from build123d import *

# Parameters (mm, degrees)
EXTRUDE_1_DEPTH     = 20
SKETCH_2_R          = 1.5
CUT_EXTRUDE_1_DEPTH = 20


with BuildPart() as part:
    # 草图1 → 凸台-拉伸1 (new body)
    with BuildSketch(Plane.XY):
        with BuildLine():
            Line((-3, 20), (-3, 10.583005244))
            ThreePointArc((-3, 10.583005244), (-11, 0), (-3, -10.583005244))
            Line((-3, -10.583005244), (-3, -45.2))
            Line((-3, -45.2), (0, -45.2))
            Line((0, -45.2), (0, -10))
            ThreePointArc((0, -10), (-10, 0), (0, 10))
            Line((0, 10), (0, 20))
            Line((0, 20), (-3, 20))
        make_face()
    extrude(amount=EXTRUDE_1_DEPTH)

    # 草图2 → 切除-拉伸1 (cut)
    with BuildSketch(Plane.ZY.offset(3)):
        with Locations((5, 15.291502622)):
            Circle(SKETCH_2_R)
        with Locations((15, 15.291502622)):
            Circle(SKETCH_2_R)
        with Locations((5, -25.7)):
            Circle(SKETCH_2_R)
        with Locations((15, -25.7)):
            Circle(SKETCH_2_R)
    extrude(amount=-CUT_EXTRUDE_1_DEPTH, mode=Mode.SUBTRACT)


solid = part.part
Part model, mm, in its own coordinate system. A direction names the side the tool comes from. Coordinates: 2 decimals unless noted, no trailing zeros. Loops run counter-clockwise (first coordinate to the right, second up) from the corner with the lowest first, then second, coordinate; pieces in that order, holes last. Notation, with made-up numbers: M 86,-22 L 116,-22 A16 cw 116,-3 Z; hole C 38.5,69 d4. An arc over 180 degrees is marked long. Use a Markdown table: item, result. Add a question column.
Q1. Mould opens along Y. For faces 4 (the flat face through (-2, -15, 20)), 5 (the cylindrical face through (-10, 0, 10)), 6 (the flat face through (-1, 20, 10)) say: +Y half, -Y half, draft (parallel to the pull), parting line (faces both ways), or undercut.
Q2. Pin check, flat tips, straight feed: P1, Ø5, axis at x = -7.5, z = 6, coming from the +Y side; P2, Ø2.5, axis at y = 15.29, z = 15, coming from the -X side; P3, Ø1.5, axis at y = -25, z = 15.5, coming from the -X side. Stop position of each tip, or through.
Q3. Cut at D-D (z = 8). Write the cut outline in (x, y).
Q4. Cut at A-A (y = -25.7). Write the cut outline in (x, z).
Q5. Cut at B-B (z = 15). Write the cut outline in (x, y), and give its area (3 significant figures).
Q6. Probe L1, parallel to Z at x = -1.75, y = -25.5; L2, parallel to Y at x = -4.5, z = 17.75; L3, parallel to Y at x = -4.25, z = 17. List the from-to ranges inside material, lowest first.
Q7. Cut at C-C (x = -7). Write the cut outline in (y, z), and give its area (3 significant figures).
Q8. Which spindle directions (+Z, -Z, +X, -X, +Y, -Y) get a long thin tool onto all of the face, cutting with end or side? Do faces 1 (the flat face through (-3, 15, 10)), 2 (the flat face through (-3, -28, 10)), 3 (the cylindrical face through (-1.521, 16.305, 13.894)). Say none if no direction does.
Worked out:
| question | item | result |
|---|---|---|
| 1 | face 4 | draft |
| 1 | face 5 | undercut |
| 1 | face 6 | +Y half |
| 2 | P1 | stops at y = 9.8 |
| 2 | P2 | passes through |
| 2 | P3 | stops at x = -3 |
| 3 | outline | M -3,-45.2 L 0,-45.2 L 0,-10 A10 cw 0,10 L 0,20 L -3,20 L -3,10.58 A11 ccw -3,-10.58 Z |
| 4 | outline | M -3,0 L 0,0 L 0,3.5 L -3,3.5 Z; M -3,6.5 L 0,6.5 L 0,13.5 L -3,13.5 Z; M -3,16.5 L 0,16.5 L 0,20 L -3,20 Z |
| 5 | outline | M -3,-45.2 L 0,-45.2 L 0,-27.2 L -3,-27.2 Z; M -3,-24.2 L 0,-24.2 L 0,-10 A10 cw 0,10 L 0,13.79 L -3,13.79 L -3,10.58 A11 ccw -3,-10.58 Z; M -3,16.79 L 0,16.79 L 0,20 L -3,20 Z |
| 5 | area | 145 mm2 |
| 6 | L1 | z = 0 to 3.51, 6.49 to 13.51, 16.49 to 20 |
| 6 | L2 | y = -10.04 to -8.93, 8.93 to 10.04 |
| 6 | L3 | y = -10.15 to -9.05, 9.05 to 10.15 |
| 7 | outline | M -8.49,0 L -7.14,0 L -7.14,20 L -8.49,20 Z; M 7.14,0 L 8.49,0 L 8.49,20 L 7.14,20 Z |
| 7 | area | 53.8 mm2 |
| 8 | face 1 | +Z, -Z, -X, +Y |
| 8 | face 2 | +Z, -Z, -X, -Y |
| 8 | face 3 | +X, -X |
